```python
from build123d import *

# Parameters (mm, degrees)
SKETCH4_R           = 82.49431047
SKETCH4_R_2         = 7.246642198
SKETCH4_R_3         = 6.35187519
SKETCH4_R_4         = 6.283502274
SKETCH4_R_5         = 6.278398691
BOSS_EXTRUDE1_DEPTH = 6.35


with BuildPart() as part:
    # Sketch4 → Boss-Extrude1 (new body)
    with BuildSketch(Plane(origin=(0, 0, 0), x_dir=(1, 0, 0), z_dir=(0, 1, 0))):
        with BuildLine():
            Line((-102.682677734, -127), (102.682677734, -127))
            ThreePointArc((102.682677734, -127), (107.172805794, -125.140128061), (109.032677734, -120.65))
            Line((109.032677734, -120.65), (109.032677734, 0))
            ThreePointArc((109.032677734, 0), (0, 109.032677734), (-109.032677734, 0))
            Line((-109.032677734, 0), (-109.032677734, -120.65))
            ThreePointArc((-109.032677734, -120.65), (-107.172805794, -125.140128061), (-102.682677734, -127))
        make_face()
        Circle(SKETCH4_R, mode=Mode.SUBTRACT)
        with Locations((-51.514938753, -115.487351309)):
            Circle(SKETCH4_R_2, mode=Mode.SUBTRACT)
        with Locations((51.514938753, -115.487351309)):
            Circle(SKETCH4_R_2, mode=Mode.SUBTRACT)
        with Locations((-93.682436309, -12.561067561)):
            Circle(SKETCH4_R_3, mode=Mode.SUBTRACT)
        with Locations((37.802843995, 87.500493595)):
            Circle(SKETCH4_R_4, mode=Mode.SUBTRACT)
        with Locations((58.697357769, -76.319875304)):
            Circle(SKETCH4_R_5, mode=Mode.SUBTRACT)
    extrude(amount=BOSS_EXTRUDE1_DEPTH)


solid = part.part
```
Verification items for the finished model (mm, model axes). Give positions to 0.01 mm unless a question says otherwise; leave off trailing zeros. Order: outer loops, then holes, each group sorted by start corner. A loop starts at its lowest first (then second) coordinate and runs counter-clockwise, first axis right, second up. Notation, with made-up numbers: (-25.5, 80) - (12.5, 80) arc R20 cw to (12.5, 112) - close; hole circle Ø5 at (75.5, -38.5). An arc over 180 degrees is marked (long way). Answer as CSV lines item,"result". Start each with the question number.
Item 1: Section check D-D, the plane x = 39.5. Record the boundary of the cut face in (y, z), plus the area to 3 significant figures.
Item 2: Section check B-B, the plane z = -30. Record the boundary of the cut face in (x, y).
Item 3: Mould release check, pull along Z, two halves, no side actions. Record for faces 1 (the face through (54.859, 3.131, 121.916)), 2 (the face through (2.398, 3.131, -109.006)), 3 (the face through (-107.22, 3.13, 125.09)): released by +Z, released by -Z, zero draft, split by the parting line, or undercut.
Item 4: Gauge pin test, flat end, axial feed: pin 1 (19 mm diameter, centred on x = -51.51, z = 115.49, fed in from +Y). Record the tip position at first contact, or that the pin passes through.
Item 5: Material ranges on L1, parallel to Z at x = 54, y = 3.5; L2, parallel to Z at x = -57, y = 3; L3, parallel to Z at x = 34, y = 0.75, recorded low to high.
Item 6: Section check C-C, the plane y = 2.5. Record the boundary of the cut face in (x, z), plus the area to 3 significant figures.
Item 7: Section check A-A, the plane x = 0. Record the boundary of the cut face in (y, z), plus the area to 3 significant figures.
Filled in:
1,outline,"(0, -101.63) - (6.35, -101.63) - (6.35, -93.55) - (0, -93.55) - close; (0, -81.45) - (6.35, -81.45) - (6.35, -72.42) - (0, -72.42) - close; (0, 72.42) - (6.35, 72.42) - (6.35, 127) - (0, 127) - close"
1,area,"455 mm^2"
2,outline,"(-104.82, 0) - (-76.85, 0) - (-76.85, 6.35) - (-104.82, 6.35) - close; (76.85, 0) - (104.82, 0) - (104.82, 6.35) - (76.85, 6.35) - close"
3,face 1,"undercut"
3,face 2,"released by -Z"
3,face 3,"released by +Z"
4,pin 1,"y = 6.35"
5,L1,"-94.72 to -62.36, 62.36 to 72.15, 80.49 to 108.68, 122.29 to 127"
5,L2,"-92.95 to -59.63, 59.63 to 110.75, 120.22 to 127"
5,L3,"-103.6 to -92.5, -82.5 to -75.16, 75.16 to 127"
6,outline,"(-109.03, 0) arc R109.03 ccw to (109.03, 0) - (109.03, 120.65) arc R6.35 ccw to (102.68, 127) - (-102.68, 127) arc R6.35 ccw to (-109.03, 120.65) - close; hole circle Ø12.7 at (-93.68, 12.56); hole circle Ø164.99 at (0, 0); hole circle Ø14.49 at (-51.51, 115.49); hole circle Ø12.57 at (37.8, -87.5); hole circle Ø14.49 at (51.51, 115.49); hole circle Ø12.56 at (58.7, 76.32)"
6,area,"24,300 mm^2"
7,outline,"(0, -109.03) - (6.35, -109.03) - (6.35, -82.49) - (0, -82.49) - close; (0, 82.49) - (6.35, 82.49) - (6.35, 127) - (0, 127) - close"
7,area,"451 mm^2"
